Verification items for the finished model (mm, model axes). A direction names the side the tool comes from. Coordinates: 2 decimals unless noted, no trailing zeros. Order: outer loops, then holes, each group sorted by start corner. A loop starts at its lowest first (then second) coordinate and runs counter-clockwise, first axis right, second up. Notation, with made-up numbers: (82.5, -19) -> (93.5, -19) arc R33 ccw to (93.5, 12) -> close; hole circle Ø7 at (53.25, 52.25). An arc over 180 degrees is marked (long way). Write each question's results on one line, items separated by ' | '. Start each with the question number.
(1) Cross-section at A-A on z = -6. Give the number of separate pieces and of enclosed holes in the cut face, and give its area (3 significant figures).
(2) Thickness scan on probe 1 along Y at (x, z) = (-40, -13.5); probe 2 along Y at (x, z) = (38, -3); probe 3 along Z at (x, y) = (46, 10.5). Record the ranges inside material, lowest first. Write a range as [from, to].
(3) Go/stop test with flat-tipped pins: pin 1 (4 mm diameter, centred on y = -14, z = -12, fed in from +X); pin 2 (2.5 mm diameter, centred on x = 43.5, z = -15, fed in from +Y); pin 3 (6.5 mm diameter, centred on x = -68, y = 15.5, fed in from +Z); pin 4 (9.5 mm diameter, centred on y = -3.5, z = -15.5, fed in from -X). Record where each tip stops, or that it passes through.
(4) Draft check along Y on faces 1 (the flat face through (1, 24, -10)), 2 (the flat face through (1, 26, -20)), 3 (the conical face through (74.635, -22.026, -19.493)). Enter one of: +Y half, -Y half, draft (parallel to the pull), parting line (faces both ways), or undercut.
(5) Set-up check for faces 4 (the conical face through (-74.635, -22.046, -8.507)), 5 (the flat face through (1, -26, -20)), 6 (the cylindrical face through (-49.185, 1.201, -3.944)): record each of +Z, -Z, +X, -X, +Y, -Y from which the full face is reachable in a straight line by a thin tool's end or side.
(6) Cross-section at B-B on x = 6.5. Enter the section's corners in (y, z).
```python
from build123d import *

# Parameters (mm, degrees)
F0_W     = 150
F0_H     = 58
F1_DEPTH = 29
F3_W     = 5
F3_H     = 20
F4_DEPTH = 150.001
F2_R     = 4
F5_DEPTH = 20
F8_DEPTH = 50
F9_DEPTH = 50
F10_SIZE = 0.5


with BuildPart() as f1:
    # F0 (on Top) → F1 (new body)
    with BuildSketch(Plane.XY):
        Rectangle(F0_W, F0_H)
    extrude(amount=-F1_DEPTH)

    # F3 (on face) → F4 (cut, through all)
    with BuildSketch(Plane.YZ.offset(75)):
        with Locations((-26.5, -10)):
            Rectangle(F3_W, F3_H)
        with Locations((26.5, -10)):
            Rectangle(F3_W, F3_H)
    extrude(amount=-F4_DEPTH, mode=Mode.SUBTRACT)

    # F2 (on Top) → F5 (cut)
    with BuildSketch(Plane.XY):
        with Locations((68, 15.5)):
            Circle(F2_R)
        with Locations((38, -15.5)):
            Circle(F2_R)
        with Locations((38, 15.5)):
            Circle(F2_R)
        with Locations((38, 0)):
            Circle(F2_R)
        with Locations((68, 0)):
            Circle(F2_R)
        with Locations((53, -15.5)):
            Circle(F2_R)
        with Locations((68, -15.5)):
            Circle(F2_R)
        with Locations((53, 0)):
            Circle(F2_R)
        with Locations((53, 15.5)):
            Circle(F2_R)
        with Locations((-68, 15.5)):
            Circle(F2_R)
        with Locations((-53, 0)):
            Circle(F2_R)
        with Locations((-38, 0)):
            Circle(F2_R)
        with Locations((-68, -15.5)):
            Circle(F2_R)
        with Locations((-38, -15.5)):
            Circle(F2_R)
        with Locations((-68, 0)):
            Circle(F2_R)
        with Locations((-38, 15.5)):
            Circle(F2_R)
        with Locations((-53, 15.5)):
            Circle(F2_R)
        with Locations((-53, -15.5)):
            Circle(F2_R)
    extrude(amount=-F5_DEPTH, mode=Mode.SUBTRACT)

    # F6 (on face) → F8 (cut)
    with BuildSketch(Plane.YZ.offset(75)):
        with BuildLine():
            Line((-10.5, -8), (-20.5, -8))
            ThreePointArc((-20.5, -8), (-21.9142135624, -8.5857864376), (-22.5, -10))
            Line((-22.5, -10), (-22.5, -18))
            ThreePointArc((-22.5, -18), (-21.9142135624, -19.4142135624), (-20.5, -20))
            Line((-20.5, -20), (-10.5, -20))
            ThreePointArc((-10.5, -20), (-9.0857864376, -19.4142135624), (-8.5, -18))
            Line((-8.5, -18), (-8.5, -10))
            ThreePointArc((-8.5, -10), (-9.0857864376, -8.5857864376), (-10.5, -8))
        make_face()
        with BuildLine():
            Line((7, -18), (7, -10))
            ThreePointArc((7, -10), (6.4142135624, -8.5857864376), (5, -8))
            Line((5, -8), (-5, -8))
            ThreePointArc((-5, -8), (-6.4142135624, -8.5857864376), (-7, -10))
            Line((-7, -10), (-7, -18))
            ThreePointArc((-7, -18), (-6.4142135624, -19.4142135624), (-5, -20))
            Line((-5, -20), (5, -20))
            ThreePointArc((5, -20), (6.4142135624, -19.4142135624), (7, -18))
        make_face()
        with BuildLine():
            Line((22.5, -18), (22.5, -10))
            ThreePointArc((22.5, -10), (21.9142135624, -8.5857864376), (20.5, -8))
            Line((20.5, -8), (10.5, -8))
            ThreePointArc((10.5, -8), (9.0857864376, -8.5857864376), (8.5, -10))
            Line((8.5, -10), (8.5, -18))
            ThreePointArc((8.5, -18), (9.0857864376, -19.4142135624), (10.5, -20))
            Line((10.5, -20), (20.5, -20))
            ThreePointArc((20.5, -20), (21.9142135624, -19.4142135624), (22.5, -18))
        make_face()
    extrude(amount=-F8_DEPTH, mode=Mode.SUBTRACT)

    # F7 (on face) → F9 (cut)
    with BuildSketch(Plane(origin=(-75, 0, 0), x_dir=(0, -1, 0), z_dir=(-1, 0, 0))):
        with BuildLine():
            Line((-10.4802631579, -8), (-20.4802631579, -8))
            ThreePointArc((-20.4802631579, -8), (-21.8944767203, -8.5857864376), (-22.4802631579, -10))
            Line((-22.4802631579, -10), (-22.4802631579, -18))
            ThreePointArc((-22.4802631579, -18), (-21.8944767203, -19.4142135624), (-20.4802631579, -20))
            Line((-20.4802631579, -20), (-10.4802631579, -20))
            ThreePointArc((-10.4802631579, -20), (-9.0660495955, -19.4142135624), (-8.4802631579, -18))
            Line((-8.4802631579, -18), (-8.4802631579, -10))
            ThreePointArc((-8.4802631579, -10), (-9.0660495955, -8.5857864376), (-10.4802631579, -8))
        make_face()
        with BuildLine():
            Line((7.0197368421, -18), (7.0197368421, -10))
            ThreePointArc((7.0197368421, -10), (6.4339504045, -8.5857864376), (5.0197368421, -8))
            Line((5.0197368421, -8), (-4.9802631579, -8))
            ThreePointArc((-4.9802631579, -8), (-6.3944767203, -8.5857864376), (-6.9802631579, -10))
            Line((-6.9802631579, -10), (-6.9802631579, -18))
            ThreePointArc((-6.9802631579, -18), (-6.3944767203, -19.4142135624), (-4.9802631579, -20))
            Line((-4.9802631579, -20), (5.0197368421, -20))
            ThreePointArc((5.0197368421, -20), (6.4339504045, -19.4142135624), (7.0197368421, -18))
        make_face()
        with BuildLine():
            Line((22.5197368421, -18), (22.5197368421, -10))
            ThreePointArc((22.5197368421, -10), (21.9339504045, -8.5857864376), (20.5197368421, -8))
            Line((20.5197368421, -8), (10.5197368421, -8))
            ThreePointArc((10.5197368421, -8), (9.1055232797, -8.5857864376), (8.5197368421, -10))
            Line((8.5197368421, -10), (8.5197368421, -18))
            ThreePointArc((8.5197368421, -18), (9.1055232797, -19.4142135624), (10.5197368421, -20))
            Line((10.5197368421, -20), (20.5197368421, -20))
            ThreePointArc((20.5197368421, -20), (21.9339504045, -19.4142135624), (22.5197368421, -18))
        make_face()
    extrude(amount=-F9_DEPTH, mode=Mode.SUBTRACT)

    # F10
    f10_edges = [f1.edges().sort_by_distance(p)[0] for p in [
        (75, -15.5, -8),
        (75, 0, -8),
        (75, 15.5, -8),
        (-75, 15.480263, -8),
        (-75, -0.019737, -8),
        (-75, -15.519737, -8),
        (75, -24, -10),
        (75, 0, 0),
        (75, 24, -10),
        (0, -24, 0),
        (0, 24, 0),
        (-75, 0, 0),
        (-75, 24, -10),
        (-75, -24, -10),
        (75, -26.5, -20),
        (0, -29, -20),
        (-75, -26.5, -20),
        (75, 26.5, -20),
        (0, 29, -20),
        (-75, 26.5, -20),
        (75, 29, -24.5),
        (75, -29, -24.5),
        (-75, 29, -24.5),
        (-75, -29, -24.5),
        (0, -29, -29),
        (-75, 0, -29),
        (75, 0, -29),
        (0, 29, -29),
    ]]
    chamfer(f10_edges, length=F10_SIZE)


solid = f1.part
```
Results are:
1) separate pieces: 1 | enclosed holes: 18 | area: 6,290 mm2
2) probe 1: y = [-24, -22.52], [-8.52, -7.02], [6.98, 8.48], [22.48, 24] | probe 2: y = [-24, -19.5], [-11.5, -4], [4, 11.5], [19.5, 24] | probe 3: z = [-29, -20], [-8, 0]
3) pin 1: stops at x = 25 | pin 2: stops at y = 24 | pin 3: stops at z = -20 | pin 4: stops at x = -75
4) face 1: +Y half | face 2: draft | face 3: undercut
5) face 4: -X | face 5: +Z, +X, -X, -Y | face 6: +Z
6) outline: (-29, -28.5) -> (-28.5, -29) -> (28.5, -29) -> (29, -28.5) -> (29, -20.5) -> (28.5, -20) -> (24, -20) -> (24, -0.5) -> (23.5, 0) -> (-23.5, 0) -> (-24, -0.5) -> (-24, -20) -> (-28.5, -20) -> (-29, -20.5) -> close
